from build123d import *

# Parameters (mm, degrees)
CROQUIS1_R              = 75
SALIENTE_EXTRUIR1_DEPTH = 5
CORTAR_EXTRUIR1_DEPTH   = 5
CORTAR_EXTRUIR2_DEPTH   = 5
CROQUIS6_R              = 4.5
CROQUIS11_W             = 43
CROQUIS11_H             = 3
CORTAR_EXTRUIR3_DEPTH   = 5
CROQUIS12_R             = 2
CORTAR_EXTRUIR4_DEPTH   = 5


with BuildPart() as part:
    # Croquis1 → Saliente-Extruir1 (new body)
    with BuildSketch(Plane(origin=(0, 0, 0), x_dir=(1, 0, 0), z_dir=(0, 1, 0))):
        with Locations(Location((0, 0, 0), (0, 0, 270))):
            Circle(CROQUIS1_R)
    extrude(amount=SALIENTE_EXTRUIR1_DEPTH)

    # Croquis2 → Cortar-Extruir1 (cut)
    with BuildSketch(Plane(origin=(0, 5, 0), x_dir=(1, 0, 0), z_dir=(0, 1, 0))):
        Polygon((31, 0), (0, 0), (-12, 0), (-12, -13), (31, -13), align=None)
        Polygon((-12, 0), (0, 0), (31, 0), (31, 13), (-12, 13), align=None)
    extrude(amount=-CORTAR_EXTRUIR1_DEPTH, mode=Mode.SUBTRACT)

    # Croquis4 → Cortar-Extruir2 (cut)
    with BuildSketch(Plane(origin=(0, 5, 0), x_dir=(1, 0, 0), z_dir=(0, 1, 0))):
        with BuildLine():
            ThreePointArc((-28.5, 30), (-31.060660172, 31.060660172), (-30, 28.5))
            Line((-30, 28.5), (-30, 30))
            Line((-30, 30), (-28.5, 30))
        make_face()
        with BuildLine():
            Line((-30, 30), (-30, 28.5))
            ThreePointArc((-30, 28.5), (-28.939339828, 28.939339828), (-28.5, 30))
            Line((-28.5, 30), (-30, 30))
        make_face()
        with BuildLine():
            ThreePointArc((28.5, 30), (28.939339828, 28.939339828), (30, 28.5))
            Line((30, 28.5), (30, 30))
            Line((30, 30), (28.5, 30))
        make_face()
        with BuildLine():
            Line((30, 30), (30, 28.5))
            ThreePointArc((30, 28.5), (31.060660172, 28.939339828), (31.5, 30))
            ThreePointArc((31.5, 30), (30, 31.5), (28.5, 30))
            Line((28.5, 30), (30, 30))
        make_face()
        with BuildLine():
            ThreePointArc((30, -28.5), (28.939339828, -28.939339828), (28.5, -30))
            Line((28.5, -30), (30, -30))
            Line((30, -30), (30, -28.5))
        make_face()
        with BuildLine():
            Line((30, -30), (28.5, -30))
            ThreePointArc((28.5, -30), (30, -31.5), (31.5, -30))
            ThreePointArc((31.5, -30), (31.060660172, -28.939339828), (30, -28.5))
            Line((30, -28.5), (30, -30))
        make_face()
        with BuildLine():
            Line((-30, -28.5), (-30, -30))
            Line((-30, -30), (-28.5, -30))
            ThreePointArc((-28.5, -30), (-28.939339828, -28.939339828), (-30, -28.5))
        make_face()
        with BuildLine():
            Line((-28.5, -30), (-30, -30))
            Line((-30, -30), (-30, -28.5))
            ThreePointArc((-30, -28.5), (-31.060660172, -31.060660172), (-28.5, -30))
        make_face()
    extrude(amount=-CORTAR_EXTRUIR2_DEPTH, mode=Mode.SUBTRACT)

    # Cortar-Barrer3: sweep along a path in Croquis5
    with BuildLine(Plane(origin=(0, 5, 0), x_dir=(1, 0, 0), z_dir=(0, 1, 0))) as cortar_barrer3_path:
        CenterArc((0, 0), 64.5, 0, 360)
    # Croquis6 → Cortar-Barrer3 (sweep, cut)
    with BuildSketch(Plane.XY):
        with Locations((64.5, 8)):
            Circle(CROQUIS6_R)
    sweep(path=cortar_barrer3_path.line, mode=Mode.SUBTRACT)

    # Croquis11 → Cortar-Extruir3 (cut)
    with BuildSketch(Plane(origin=(0, 5, 0), x_dir=(1, 0, 0), z_dir=(0, 1, 0))):
        with Locations((9.5, 14.5)):
            Rectangle(CROQUIS11_W, CROQUIS11_H)
        with Locations((9.5, -14.5)):
            Rectangle(CROQUIS11_W, CROQUIS11_H)
    extrude(amount=-CORTAR_EXTRUIR3_DEPTH, mode=Mode.SUBTRACT)

    # Croquis12 → Cortar-Extruir4 (cut)
    with BuildSketch(Plane(origin=(0, 5, 0), x_dir=(1, 0, 0), z_dir=(0, 1, 0))):
        with Locations(Location((34.8, 5, 0), (0, 0, 270))):
            Circle(CROQUIS12_R)
        with Locations(Location((34.8, -5, 0), (0, 0, 270))):
            Circle(CROQUIS12_R)
        with Locations(Location((-15.8, -5, 0), (0, 0, 270))):
            Circle(CROQUIS12_R)
        with Locations(Location((-15.8, 5, 0), (0, 0, 270))):
            Circle(CROQUIS12_R)
    extrude(amount=-CORTAR_EXTRUIR4_DEPTH, mode=Mode.SUBTRACT)


solid = part.part
Source: CAD feature listing. Evaluate the final solid. Frame: model axes, mm. A direction names the side the tool comes from. Coordinates: 2 decimals unless noted, no trailing zeros. Write each loop counter-clockwise with the first axis right and the second up, starting at its lowest first coordinate (ties: lowest second). Pieces come first, ordered by that corner, then holes. Notation, with made-up numbers: M 2.25,-30 L 20.25,-30 A26 ccw 20.25,3 Z; hole C 77.25,33 d10. An arc over 180 degrees is marked long. Use a Markdown table: item, result.
1) Section C-C, the plane y = 2.6. Give the number of separate pieces and of enclosed holes in the cut face, then the cut area to 3 significant figures.
Conclusion:
| item | result |
|---|---|
| separate pieces | 1 |
| enclosed holes | 9 |
| area | 16,200 mm^2 |
2) Section A-A, the plane x = 0. Output: boundary loops of the cut face in (y, z), then the cut area to 3 significant figures.
Conclusion:
| item | result |
|---|---|
| outline | M 0,-75 L 5,-75 L 5,-67.85 A4.5 cw 5,-61.15 L 5,-16 L 0,-16 Z; M 0,16 L 5,16 L 5,61.15 A4.5 cw 5,67.85 L 5,75 L 0,75 Z |
| area | 576 mm^2 |
3) Mould query, pull axis Z, two halves, no side actions, for faces 1 (the flat face through (31, 3, 0)), 2 (the cylindrical face through (-17.752, 2.535, -5.434)), 3 (the flat face through (-13, 5, -1)), 4 (the cylindrical face through (-45.636, 2.465, -59.517)). Classes: pulls with the +Z half, pulls with the -Z half, needs draft (parallel to the pull), parting line crosses it, or undercut.
Conclusion:
| item | result |
|---|---|
| face 1 | undercut |
| face 2 | undercut |
| face 3 | needs draft |
| face 4 | parting line crosses it |
4) First-contact query: pin 1 Ø4.5 at (x, z) = (34.8, -5) entering from -Y; pin 2 Ø1 at (y, z) = (2, 24) entering from -X; pin 3 Ø2.5 at (x, y) = (8.5, 1.5) entering from +Z; pin 4 Ø3 at (x, y) = (-24.5, 0.5) entering from +Z. Flat tips, straight axial feed; report the tip coordinate or a pass-through.
Conclusion:
| item | result |
|---|---|
| pin 1 | stops at y = 0 |
| pin 2 | stops at x = -71.22 |
| pin 3 | stops at z = 74.65 |
| pin 4 | stops at z = 71.39 |
5) Reachability of faces 5 (the flat face through (-39, 5, -56)), 6 (the flat face through (9, 3, 16)) from +Z, -Z, +X, -X, +Y, -Y: full face, straight path, thin tool, end or side. Return the list, or none.
Conclusion:
| item | result |
|---|---|
| face 5 | +Z, -Z, +X, -X, +Y |
| face 6 | +Y, -Y |
6) Ray query, L1, parallel to X at y = 3.9, z = 5; L2, parallel to X at y = 3.85, z = 5; L3, parallel to X at y = 1.45, z = 5. Return the intervals inside material, ascending.
Conclusion:
| item | result |
|---|---|
| L1 | x = -74.83 to -66.17, -62.45 to -17.8, -13.8 to -12, 31 to 32.8, 36.8 to 62.45, 66.17 to 74.83 |
| L2 | x = -74.83 to -66.05, -62.56 to -17.8, -13.8 to -12, 31 to 32.8, 36.8 to 62.56, 66.05 to 74.83 |
| L3 | x = -74.83 to -17.8, -13.8 to -12, 31 to 32.8, 36.8 to 74.83 |
7) Section B-B, the plane z = 0. Output: boundary loops of the cut face in (x, y), then the cut area to 3 significant figures.
Conclusion:
| item | result |
|---|---|
| outline | M -75,0 L -12,0 L -12,5 L -61.15,5 A4.5 cw -67.85,5 L -75,5 Z; M 31,0 L 75,0 L 75,5 L 67.85,5 A4.5 cw 61.15,5 L 31,5 Z |
| area | 521 mm^2 |
